Geometry: see drawing. Coordinates: mm, zero at the bounding-box minimum. Round coordinates to 2 decimals unless told otherwise and drop trailing zeros. Loops run counter-clockwise (first coordinate to the right, second up) from the corner with the lowest first, then second, coordinate; pieces in that order, holes last. Notation, with made-up numbers: (-12, -23.75) - (22, -23.75) arc R18 ccw to (22, 11.25) - close; hole circle Ø10 at (89.5, -0.5). An arc over 180 degrees is marked (long way). Answer in a Markdown table with one row per item. Add a question column.
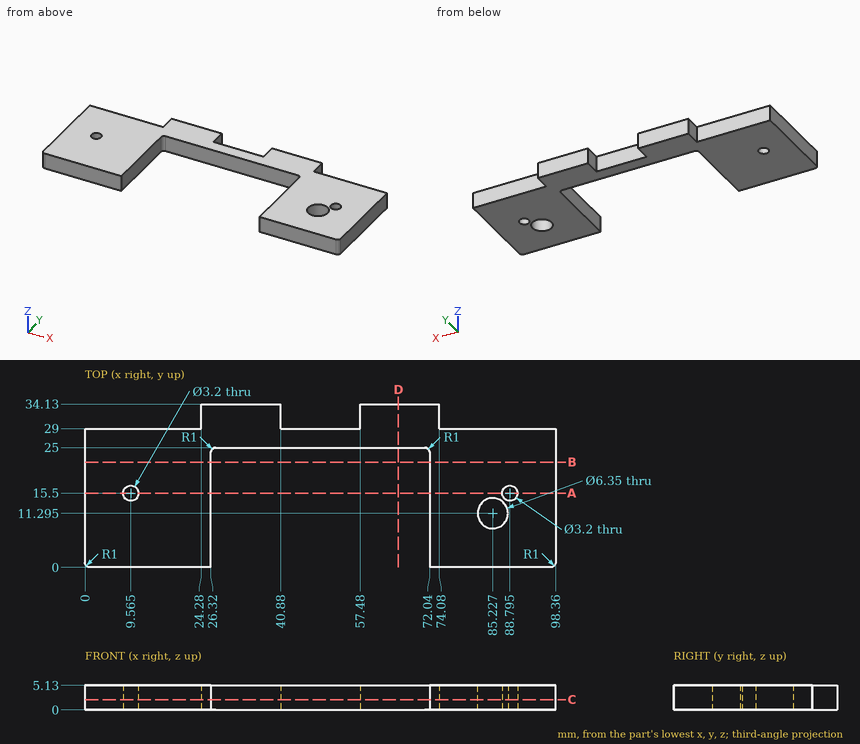
1) Contact query for flat-ended pins moving along their axis: pin 1 Ø2.5 at (y, z) = (32, 2) entering from -X; pin 2 Ø2.5 at (x, y) = (9.565, 15.5) entering from -Z (3 decimals); pin 3 Ø2.5 at (y, z) = (32, 2.5) entering from +X; pin 4 Ø2.5 at (x, z) = (12, 2.5) entering from +Y. Output: stop coordinate, or through.
2) Section C-C, the plane z = 2.15. Give the number of separate pieces and of enclosed holes in the cut face, and give its area (3 significant figures).
3) Section D-D, the plane x = 65.5. Return the cut outline in (y, z).
4) Section A-A, the plane y = 15.5. Return the cut outline in (x, z) (1 decimal).
5) Material intervals for line 1 along X through (y, z) = (29.5, 0.45); line 2 along X through (y, z) = (15, 3.2) (1 decimal); line 3 along X through (y, z) = (4.5, 1.5), sorted ascending. Write a range as from..to.
6) Section B-B, the plane y = 22. Return the cut outline in (x, z), and give its area (3 significant figures).
Evaluation:
| question | item | result |
|---|---|---|
| 1 | pin 1 | stops at x = 24.28 |
| 1 | pin 2 | passes through |
| 1 | pin 3 | stops at x = 74.08 |
| 1 | pin 4 | stops at y = 29 |
| 2 | separate pieces | 1 |
| 2 | enclosed holes | 3 |
| 2 | area | 1,830 mm² |
| 3 | outline | (25, 0) - (34.13, 0) - (34.13, 5.13) - (25, 5.13) - close |
| 4 | outline | (0, 0) - (8, 0) - (8, 5.1) - (0, 5.1) - close; (11.2, 0) - (26.3, 0) - (26.3, 5.1) - (11.2, 5.1) - close; (72, 0) - (87.2, 0) - (87.2, 5.1) - (72, 5.1) - close; (90.4, 0) - (98.4, 0) - (98.4, 5.1) - (90.4, 5.1) - close |
| 5 | line 1 | x = 24.28..40.88, 57.48..74.08 |
| 5 | line 2 | x = 0..8, 11.1..26.3, 72..87.3, 90.3..98.4 |
| 5 | line 3 | x = 0..26.32, 72.04..98.36 |
| 6 | outline | (0, 0) - (26.32, 0) - (26.32, 5.13) - (0, 5.13) - close; (72.04, 0) - (98.36, 0) - (98.36, 5.13) - (72.04, 5.13) - close |
| 6 | area | 270 mm² |
